The listing builds one solid part. Answer for the finished solid, in the listing's coordinates (mm). Round coordinates to 2 decimals unless told otherwise and drop trailing zeros. Write each loop counter-clockwise with the first axis right and the second up, starting at its lowest first coordinate (ties: lowest second). Pieces come first, ordered by that corner, then holes. Notation, with made-up numbers: M 82.25,13 L 98.25,13 A33 cw 98.25,44 Z; hole C 15,25 d8. An arc over 180 degrees is marked long. Write each question's results on one line, items separated by ' | '.
Autodesk Inventor part; units mm, degrees
ref_plane "YZ Plane" through (0, 0, 0) normal (1, 0, 0) x (0, 1, 0)
ref_plane "XZ Plane" through (0, 0, 0) normal (0, 1, 0) x (-1, 0, 0)
ref_plane "XY Plane" through (0, 0, 0) normal (0, 0, 1) x (1, 0, 0)
sketch "Sketch1" plane through (0, 0, 0) normal (0, 0, 1) x (1, 0, 0)
  line L0 (-4.5, -2.5) -> (4.5, -2.5)
  line L1 (4.5, -2.5) -> (4.5, 2.5)
  line L2 (4.5, 2.5) -> (-4.5, 2.5)
  line L3 (-4.5, 2.5) -> (-4.5, -2.5)
  line L4 (-4.5, -2.5) -> (4.5, 2.5) construction
  line L5 (4.5, -2.5) -> (-4.5, 2.5) construction
  point P0 (0, 0)
  dimension "d0" = 9
  dimension "d1" = 5
extrude "Extrusion1" add sketch "Sketch1" against normal blind 0.7 draft -45
fillet "Fillet1" radius 2 4 edges at (-4.15, -2.15, -0.35) (-4.15, 2.15, -0.35) (4.15, -2.15, -0.35) (4.15, 2.15, -0.35)
properties part number "Base"
1) Section B-B (y = 0.3) is taken. Determine the outline of the cut face in (x, z).
Return value:
outline: M -4.5,0 L -3.8,-0.7 L 3.8,-0.7 L 4.5,0 Z
2) Find the intervals of material crossed by line 1 (X direction, y = -0.15, z = -0.2); line 2 (X direction, y = -1.9, z = -0.1); line 3 (Y direction, x = 2.5, z = -0.55), in increasing order.
Return value:
line 1: -4.3 to 4.3 | line 2: -4.13 to 4.13 | line 3: -1.95 to 1.95
3) Section A-A (x = 2.25) is taken. Determine the outline of the cut face in (y, z), then the cut area to 3 significant figures.
Return value:
outline: M -2.5,0 L -1.8,-0.7 L 1.8,-0.7 L 2.5,0 Z | area: 3.01 mm²
4) This flat-tipped pin is pushed along its axis until it touches: pin 1 (2 mm diameter, centred on x = 3, y = -1.5, fed in from +Z). Where does it stop, or does it pass through?
Return value:
pin 1: z = 0
